Design review of the part built by this model. Coordinates are the model's own, in mm. A direction names the side the tool comes from. Coordinates: 2 decimals unless noted, no trailing zeros. Loops run counter-clockwise (first coordinate to the right, second up) from the corner with the lowest first, then second, coordinate; pieces in that order, holes last.
Q1. Machinability: for faces 1 (the face through (0, 68.5, 0)), 2 (the face through (-1.08, 0.51, 4.88)), 3 (the face through (0, 0, 0)), which of the approach directions +Z, -Z, +X, -X, +Y, -Y give a long, thin tool a straight path to every point of the face, cutting with its end or side? Answer none if there is none.
Q2. Add section A-A on x = -2.75. Give the boundary of the cut face in (y, z).
Q3. Add section C-C on y = 36.5. Give the boundary of the cut face in (x, z).
Q4. Add section B-B on z = 3.25. Give the boundary of the cut face in (x, y).
Q5. Add section D-D on x = 5.75. Give the boundary of the cut face in (y, z), and give its area (3 significant figures).
Q6. Wall thickness on probe 1 along Z at (x, y) = (0, 68.8); probe 2 along Y at (x, z) = (1.5, -6.5); probe 3 along Y at (x, z) = (2.75, 1.25): over which ranges is each line inside the solid? List them lowest first.
Q7. Draft analysis for pull direction Z (two halves, no side actions). For faces 4 (the face through (-1.08, 69.01, 4.88)), 5 (the face through (4, 1, -4)), 6 (the face through (2.01, 34.77, 9.03)), state which applies: released by +Z, released by -Z, zero draft, split by the parting line, or undercut.
Q8. For P1, Ø5, axis at x = 3.5, y = 35.5, coming from the +Z side; P2, Ø3, axis at y = 56, z = 5, coming from the -X side; P3, Ø1, axis at x = 3.5, y = 62, coming from the +Z side; P4, Ø11, axis at x = -1, z = -2, coming from the +Y side, all flat-tipped, find the tip position at first contact; note any pin that passes through.
Autodesk Inventor part; units mm, degrees
ref_plane "YZ Plane" through (0, 0, 0) normal (1, 0, 0) x (0, 1, 0)
ref_plane "XZ Plane" through (0, 0, 0) normal (0, 1, 0) x (-1, 0, 0)
ref_plane "XY Plane" through (0, 0, 0) normal (0, 0, 1) x (1, 0, 0)
sketch "스케치1" plane through (0, 0, 0) normal (0, 1, 0) x (-1, 0, 0)
  circle A0 centre (0, 0) radius 9.25
  dimension "d0" = 18.5
extrude "돌출1" add sketch "스케치1" along normal blind 69.5
sketch "스케치2" plane through (0, 69.5, 0) normal (0, 1, 0) x (1, 0, 0)
  circle A0 centre (0, 0) radius 5
  dimension "d3" = 10
extrude "돌출2" cut sketch "스케치2" against normal blind 1
sketch "스케치3" plane through (0, 0, 0) normal (0, -1, 0) x (1, 0, 0)
  circle A0 centre (0, 0) radius 9.25
extrude "돌출3" cut sketch "스케치3" against normal blind 1
sketch "스케치4" plane through (0, 1, 0) normal (0, -1, 0) x (1, 0, 0)
  circle A0 centre (0, 0) radius 5
  dimension "d8" = 10
extrude "돌출4" add sketch "스케치4" along normal blind 1
properties part number "건전지"
Entries:
1. face 1: +Y
1. face 2: -Y
1. face 3: +Z, -Z, +X, -X, -Y
2. outline: (0, -4.18) - (1, -4.18) - (1, -8.83) - (69.5, -8.83) - (69.5, -4.18) - (68.5, -4.18) - (68.5, 4.18) - (69.5, 4.18) - (69.5, 8.83) - (1, 8.83) - (1, 4.18) - (0, 4.18) - close
3. outline: circle Ø18.5 at (0, 0)
4. outline: (-8.66, 1) - (-3.8, 1) - (-3.8, 0) - (3.8, 0) - (3.8, 1) - (8.66, 1) - (8.66, 69.5) - (3.8, 69.5) - (3.8, 68.5) - (-3.8, 68.5) - (-3.8, 69.5) - (-8.66, 69.5) - close
5. outline: (1, -7.25) - (69.5, -7.25) - (69.5, 7.25) - (1, 7.25) - close
5. area: 993 mm2
6. probe 1: z = -9.25 to -5, 5 to 9.25
6. probe 2: y = 1 to 69.5
6. probe 3: y = 0 to 68.5
7. face 4: undercut
7. face 5: zero draft
7. face 6: split by the parting line
8. P1: stops at z = 9.2
8. P2: stops at x = -8.56
8. P3: stops at z = 8.75
8. P4: stops at y = 69.5
